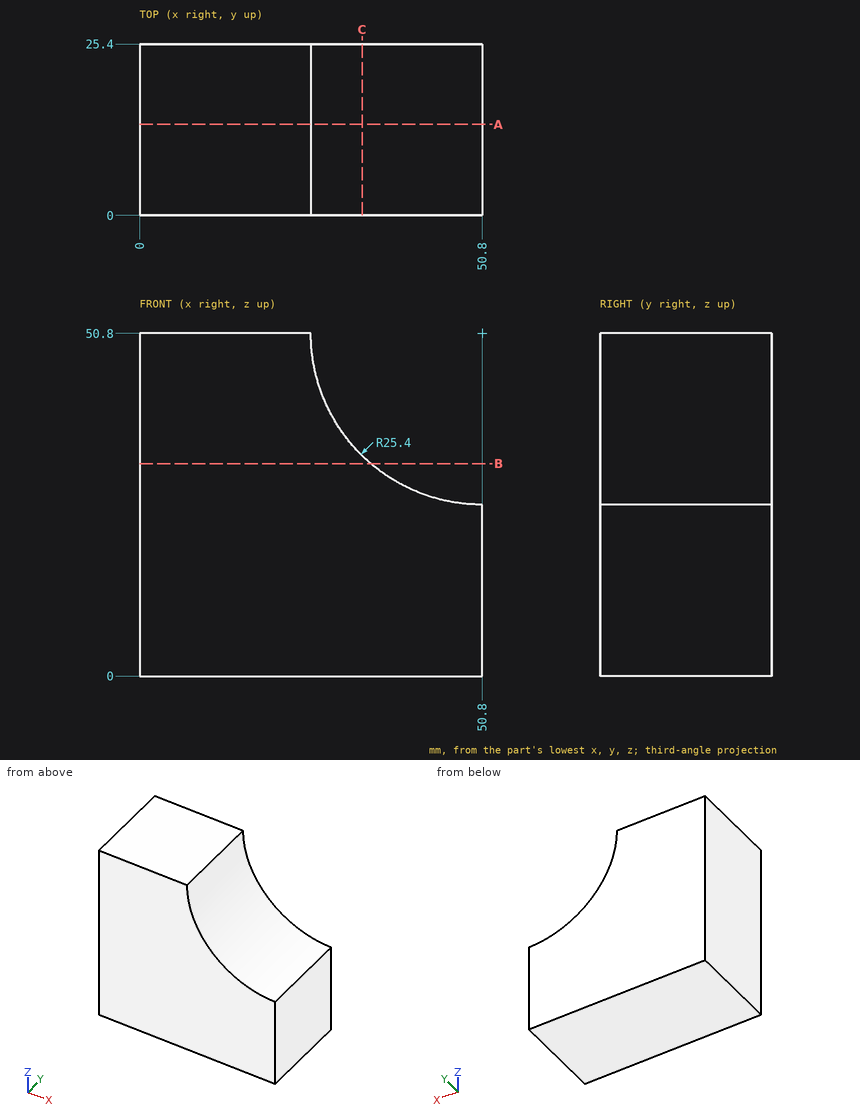
Verification items for this drawing (mm, ordinates from the low corner). Give positions to 0.01 mm unless a question says otherwise; leave off trailing zeros. Write each loop counter-clockwise with the first axis right and the second up, starting at its lowest first coordinate (ties: lowest second). Pieces come first, ordered by that corner, then holes. Notation, with made-up numbers: (7, 66.5) - (22, 66.5) arc R18 ccw to (22, 91.5) - close; hole circle Ø7 at (25, 52). An arc over 180 degrees is marked (long way). Answer as CSV lines item,"result". Start each with the question number.
1. Depth check by flat-ended pin: pin 1 (6 mm diameter, centred on y = 5.5, z = 43, fed in from +X); pin 2 (1.5 mm diameter, centred on x = 42.5, z = 29.5, fed in from -Y); pin 3 (3 mm diameter, centred on x = 35.5, y = 3.5, fed in from +Z). Enter the tip coordinate at first touch or a pass-through.
2. Thickness scan on line 1 (Z direction, x = 37, y = 24); line 2 (Z direction, x = 33.5, y = 11); line 3 (X direction, y = 17, z = 48). Record the ranges inside material, lowest first.
3. Sectioned sample at A-A (y = 13.5). Record the boundary of the cut face in (x, z), then the cut area to 3 significant figures.
4. Sectioned sample at B-B (z = 31.5). Record the boundary of the cut face in (x, y).
5. Sectioned sample at C-C (x = 33). Record the boundary of the cut face in (y, z), then the cut area to 3 significant figures.
Derived:
1,pin 1,"x = 27.81"
1,pin 2,"through"
1,pin 3,"z = 31.75"
2,line 1,"0 to 29.48"
2,line 2,"0 to 32.2"
2,line 3,"0 to 25.55"
3,outline,"(0, 0) - (50.8, 0) - (50.8, 25.4) arc R25.4 cw to (25.4, 50.8) - (0, 50.8) - close"
3,area,"2,070 mm²"
4,outline,"(0, 0) - (34.29, 0) - (34.29, 25.4) - (0, 25.4) - close"
5,outline,"(0, 0) - (25.4, 0) - (25.4, 32.68) - (0, 32.68) - close"
5,area,"830 mm²"
